Here's the drawing with two shaded views (mm, measured from the low corner). I have some questions. A direction names the side the tool comes from. Coordinates: 2 decimals unless noted, no trailing zeros. Write each loop counter-clockwise with the first axis right and the second up, starting at its lowest first coordinate (ties: lowest second). Pieces come first, ordered by that corner, then holes. Notation, with made-up numbers: (-22.75, 34.5) -> (-5.75, 34.5) arc R20 cw to (-5.75, 40.5) -> close; hole circle Ø2 at (38, -22). An arc over 180 degrees is marked (long way). Put each result on its own line as item: value.
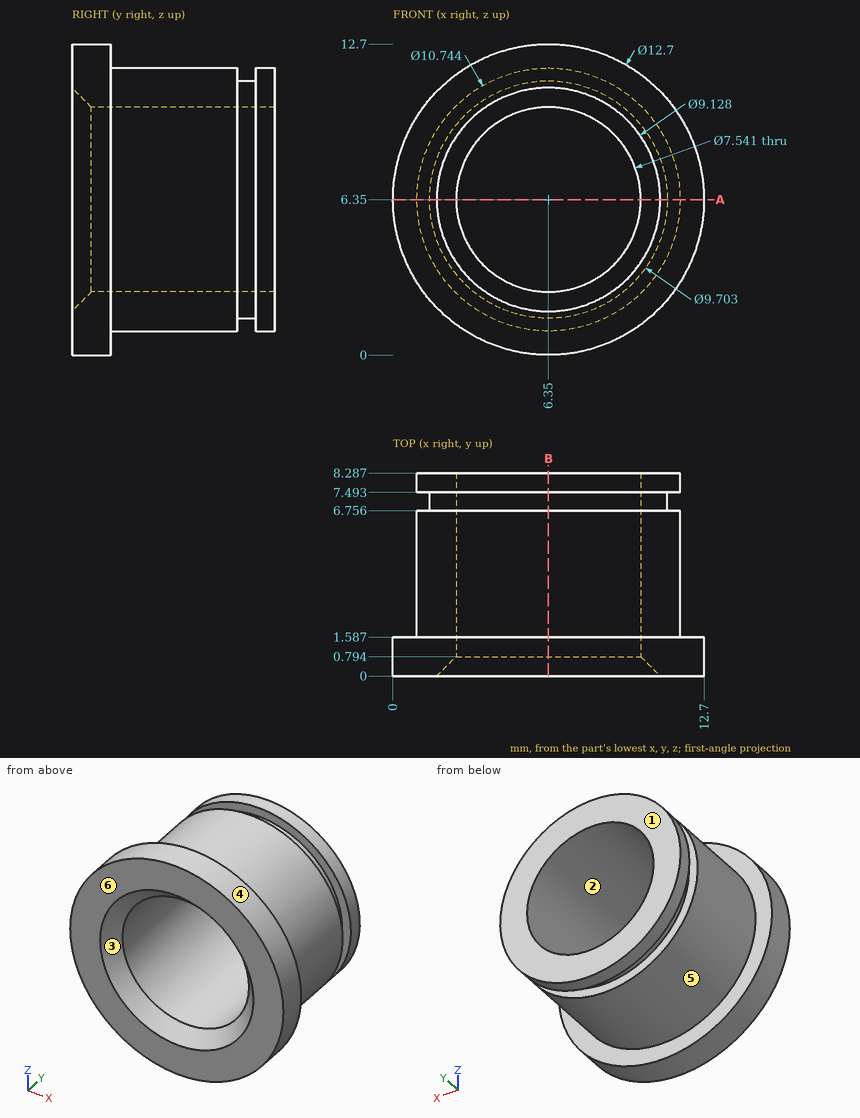
Item 1: If we mould it in two halves opening along X, with no side actions, what happens to the marked faces 1, 2, 3 and 4? For each: released by +X, released by -X, zero draft, split by the parting line, or undercut.
Output:
face 1: zero draft
face 2: undercut
face 3: undercut
face 4: split by the parting line
Item 2: Please list where these lines run through material, in increasing order: line 1 along X through (y, z) = (5.25, 6.35); line 2 along Y through (x, z) = (12.25, 8.5); line 3 along Z through (x, y) = (9, 5.5) (1 decimal). Write a range as from..to.
Output:
line 1: x = 0.98..2.58, 10.12..11.72
line 2: y = 0..1.59
line 3: z = 1.7..3.7, 9..11
Item 3: Imagine slicing it at A-A on z = 6.35. Write out the boundary of the cut face in (x, y) (1 decimal).
Output:
outline: (0, 0) -> (1.8, 0) -> (2.6, 0.8) -> (2.6, 8.3) -> (1, 8.3) -> (1, 7.5) -> (1.5, 7.5) -> (1.5, 6.8) -> (1, 6.8) -> (1, 1.6) -> (0, 1.6) -> close; (10.1, 0.8) -> (10.9, 0) -> (12.7, 0) -> (12.7, 1.6) -> (11.7, 1.6) -> (11.7, 6.8) -> (11.2, 6.8) -> (11.2, 7.5) -> (11.7, 7.5) -> (11.7, 8.3) -> (10.1, 8.3) -> close
Item 4: For P1, Ø7, axis at x = 6.35, z = 6.35, coming from the +Y side; P2, Ø3, axis at x = 7, y = 6, coming from the -Z side; P3, Ø1, axis at y = 6.5, z = 5.5, coming from the -X side, each with a flat end and sliding along its axis, tell me the tip position at first contact or that it passes through.
Output:
P1: passes through
P2: stops at z = 0.98
P3: stops at x = 0.99
Item 5: Which directions (+Z, -Z, +X, -X, +Y, -Y) give clear straight access to the entire face, cutting with the end or side of a thin tool? Please do the marked faces 5 and 6.
Output:
face 5: +Y
face 6: +Z, -Z, +X, -X, -Y
Item 6: Imagine slicing it at B-B on x = 6.35. Write out the boundary of the cut face in (y, z) (1 decimal).
Output:
outline: (0, 0) -> (1.6, 0) -> (1.6, 1) -> (6.8, 1) -> (6.8, 1.5) -> (7.5, 1.5) -> (7.5, 1) -> (8.3, 1) -> (8.3, 2.6) -> (0.8, 2.6) -> (0, 1.8) -> close; (0, 10.9) -> (0.8, 10.1) -> (8.3, 10.1) -> (8.3, 11.7) -> (7.5, 11.7) -> (7.5, 11.2) -> (6.8, 11.2) -> (6.8, 11.7) -> (1.6, 11.7) -> (1.6, 12.7) -> (0, 12.7) -> close
